The listing builds one solid part. Answer for the finished solid, in the listing's coordinates (mm). A direction names the side the tool comes from. Coordinates: 2 decimals unless noted, no trailing zeros. Loops run counter-clockwise (first coordinate to the right, second up) from the corner with the lowest first, then second, coordinate; pieces in that order, holes last. Notation, with made-up numbers: (0.5, 51.25) -> (15.5, 51.25) arc R22 ccw to (15.5, 84.25) -> close; hole circle Ø9 at (3, -8). An arc over 180 degrees is marked (long way). Answer in a Markdown table with one row per item.
```python
from build123d import *

# Parameters (mm, degrees)
SKETCH1_R           = 23
BOSS_EXTRUDE1_DEPTH = 7.5
SKETCH2_R           = 3
BOSS_EXTRUDE2_DEPTH = 10
SKETCH3_R           = 5
BOSS_EXTRUDE3_DEPTH = 10
CHAMFER1_SIZE       = 1


with BuildPart() as part:
    # Sketch1 → Boss-Extrude1 (new body)
    with BuildSketch(Plane.XY):
        Circle(SKETCH1_R)
    extrude(amount=BOSS_EXTRUDE1_DEPTH)

    # Sketch2 → Boss-Extrude2 (add)
    with BuildSketch(Plane.XY):
        with Locations((0, 17.5)):
            Circle(SKETCH2_R)
        with Locations((17.5, 0)):
            Circle(SKETCH2_R)
        with Locations((0, -17.5)):
            Circle(SKETCH2_R)
        with Locations((-17.5, 0)):
            Circle(SKETCH2_R)
    extrude(amount=-BOSS_EXTRUDE2_DEPTH)

    # Sketch3 → Boss-Extrude3 (add)
    with BuildSketch(Plane.XY.offset(7.5)):
        Circle(SKETCH3_R)
    extrude(amount=BOSS_EXTRUDE3_DEPTH)

    # Chamfer1
    chamfer1_edges = [part.edges().sort_by_distance(p)[0] for p in [
        (14.5, 0, 0),
        (-3, -17.5, 0),
        (-20.5, 0, 0),
        (-23, 0, 0),
        (-5, 0, 7.5),
        (-5, 0, 17.5),
        (-23, 0, 7.5),
        (-3, 17.5, 0),
    ]]
    chamfer(chamfer1_edges, length=CHAMFER1_SIZE)


solid = part.part
```
Item 1: A cutting plane is placed at D-D, the plane z = 11. Determine the outline of the cut face in (x, y), plus the area to 3 significant figures.
Findings below:
| item | result |
|---|---|
| outline | circle Ø10 at (0, 0) |
| area | 78.5 mm2 |
Item 2: Flat-ended cylindrical pins translate along their axes: pin 1 Ø6 at (y, z) = (-7, 10) entering from +X; pin 2 Ø8 at (x, z) = (3, 14) entering from -Y; pin 3 Ø5 at (y, z) = (0.5, -4.5) entering from -X. Find the tip coordinate at first contact, or state that the pin passes through.
Findings below:
| item | result |
|---|---|
| pin 1 | stops at x = 21.52 |
| pin 2 | stops at y = -5 |
| pin 3 | stops at x = -20.5 |
Item 3: Determine the mould class of faces 1 (the face through (15.1, -1.8, -5.4)), 2 (the face through (0, 18, -10)), 3 (the face through (-2.994, 22.804, 3.712)) for opening direction X: +X half, -X half, draft (parallel to the pull), parting line (faces both ways), or undercut.
Findings below:
| item | result |
|---|---|
| face 1 | undercut |
| face 2 | draft |
| face 3 | parting line |
Item 4: A tool of negligible diameter and unlimited length cuts with its end or side. For faces 4 (the face through (-0.65, -20.43, -5.44)), 5 (the face through (-1.08, -4.88, 12.44)), 6 (the face through (17, 0, -10)), from which of +Z, -Z, +X, -X, +Y, -Y can it reach the whole face along a straight path? Write none if from no direction.
Findings below:
| item | result |
|---|---|
| face 4 | -Z |
| face 5 | +Z |
| face 6 | -Z, +X, -X, +Y, -Y |
Item 5: A cutting plane is placed at A-A, the plane x = 0. Determine the outline of the cut face in (y, z).
Findings below:
| item | result |
|---|---|
| outline | (-23, 1) -> (-22, 0) -> (-21.5, 0) -> (-20.5, -1) -> (-20.5, -10) -> (-14.5, -10) -> (-14.5, -1) -> (-13.5, 0) -> (13.5, 0) -> (14.5, -1) -> (14.5, -10) -> (20.5, -10) -> (20.5, -1) -> (21.5, 0) -> (22, 0) -> (23, 1) -> (23, 6.5) -> (22, 7.5) -> (6, 7.5) -> (5, 8.5) -> (5, 16.5) -> (4, 17.5) -> (-4, 17.5) -> (-5, 16.5) -> (-5, 8.5) -> (-6, 7.5) -> (-22, 7.5) -> (-23, 6.5) -> close |
Item 6: Find the intervals of material crossed by probe 1 along Z at (x, y) = (-6, -3); probe 2 along Z at (x, y) = (0, 15); probe 3 along Y at (x, z) = (4, 15.5), in increasing order.
Findings below:
| item | result |
|---|---|
| probe 1 | z = 0 to 7.5 |
| probe 2 | z = -10 to 7.5 |
| probe 3 | y = -3 to 3 |
Item 7: A cutting plane is placed at C-C, the plane z = -3.25. Determine the outline of the cut face in (x, y), plus the area to 3 significant figures.
Findings below:
| item | result |
|---|---|
| outline | circle Ø6 at (-17.5, 0); circle Ø6 at (0, -17.5); circle Ø6 at (0, 17.5); circle Ø6 at (17.5, 0) |
| area | 113 mm2 |
